Here's the drawing with two shaded views (mm, measured from the low corner). I have some questions. A direction names the side the tool comes from. Round coordinates to 2 decimals unless told otherwise and drop trailing zeros. Loops run counter-clockwise (first coordinate to the right, second up) from the corner with the lowest first, then second, coordinate; pieces in that order, holes last.
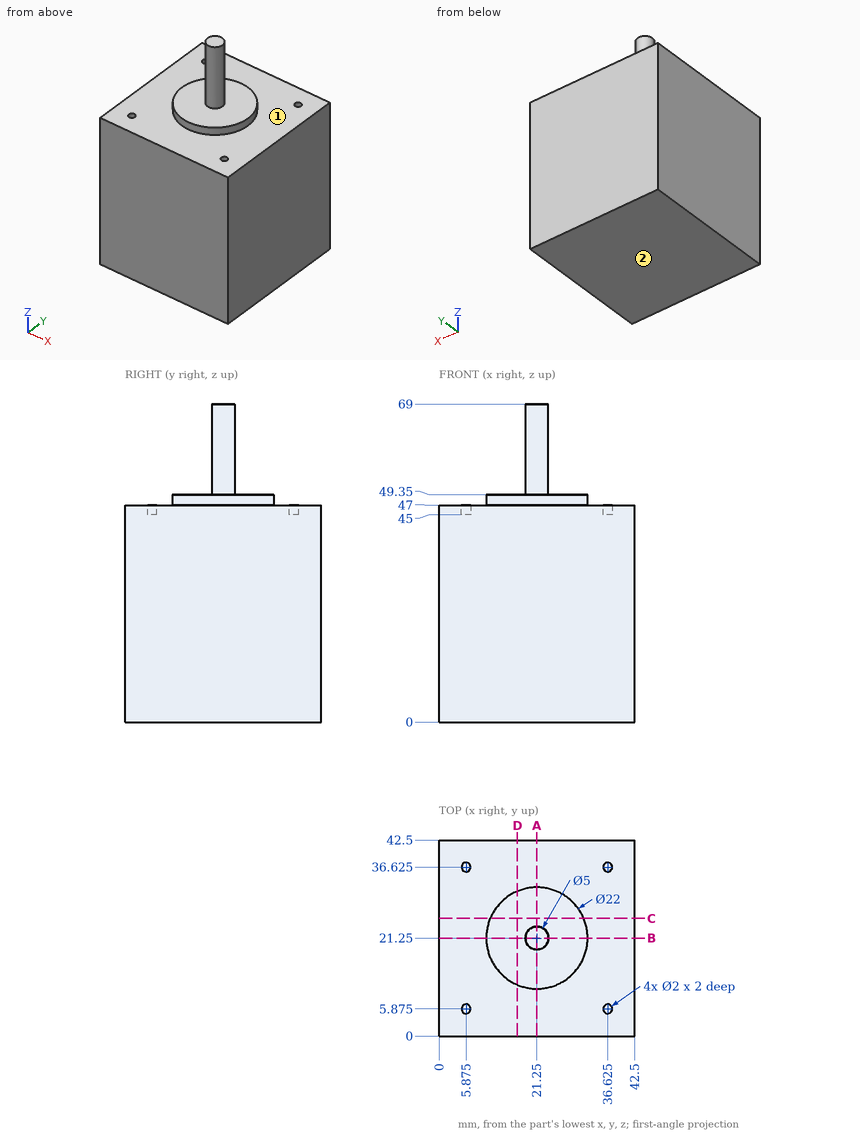
Item 1: If we section it at C-C, the plane y = 25.5: Please give me the cut outline in (x, z).
Results list:
outline: (0, 0) - (42.5, 0) - (42.5, 47) - (31.4, 47) - (31.4, 49.35) - (11.1, 49.35) - (11.1, 47) - (0, 47) - close
Item 2: If I drill on line 1 along Z through (x, y) = (10.5, 27); line 2 along Z through (x, y) = (23.5, 30.5); line 3 along X through (y, z) = (22, 65.5), over which ranges is the centre line in solid material (lowest first)?
Results list:
line 1: z = 0 to 47
line 2: z = 0 to 49.35
line 3: x = 18.87 to 23.63
Item 3: For the marked faces 1 and 2, which set-ups out of +Z, -Z, +X, -X, +Y, -Y let a thin tool reach every point of the face, with its end or its side?
Results list:
face 1: +Z
face 2: -Z, +X, -X, +Y, -Y
Item 4: If we section it at A-A, the plane x = 21.25: Please give me the cut outline in (y, z), then the cut area to 3 significant figures.
Results list:
outline: (0, 0) - (42.5, 0) - (42.5, 47) - (32.25, 47) - (32.25, 49.35) - (23.75, 49.35) - (23.75, 69) - (18.75, 69) - (18.75, 49.35) - (10.25, 49.35) - (10.25, 47) - (0, 47) - close
area: 2,150 mm2
Item 5: Will these pins go through, and if not, where does the flat tip stop? pin 1 (5 mm diameter, centred on x = 21, y = 34.5, fed in from +Z); pin 2 (1 mm diameter, centred on x = 37, y = 36.5, fed in from +Z); pin 3 (2 mm diameter, centred on x = 6, y = 5.5, fed in from +Z).
Results list:
pin 1: stops at z = 49.35
pin 2: stops at z = 45
pin 3: stops at z = 47
